Read the model definition and answer for the solid it produces. Units are mm, in the model's axes. A direction names the side the tool comes from. Coordinates: 2 decimals unless noted, no trailing zeros. Loops run counter-clockwise (first coordinate to the right, second up) from the corner with the lowest first, then second, coordinate; pieces in that order, holes last. Notation, with made-up numbers: (58.25, -21) -> (62.25, -21) arc R28 ccw to (62.25, 16) -> close; hole circle Ø3 at (89, 18). An arc over 180 degrees is marked (long way). Answer as a JSON object with one key per item and string values. Group by question number.
Q1. The part is cut by section D-D on x = 95. Write down the section's boundary in (y, z), and give its area (3 significant figures).
Q2. The part is cut by section A-A on x = 26. Write down the section's boundary in (y, z), and give its area (3 significant figures).
Q3. Determine the mould class of faces 5 (the flat face through (0, 3, 40)), 6 (the cylindrical face through (46.69, 3.2, 55.96)), 7 (the flat face through (6, 3, 0)) for opening direction X: released by +X, released by -X, zero draft, split by the parting line, or undercut.
Q4. The part is cut by section B-B on z = 49. Write down the section's boundary in (x, y), and give its area (3 significant figures).
Q5. For faces 1 (the flat face through (112.5, 3, -47)), 2 (the flat face through (122, 3, 0)), 3 (the flat face through (12, 3, 6)), 4 (the flat face through (63, 6.5, 13)), determine the directions among +Z, -Z, +X, -X, +Y, -Y from which every point of the face is accessible in a straight line to the end or side of a thin tool.
Q6. Straight lines are drawn through the part: line 1 along X through (y, z) = (5, 61); line 2 along Z through (x, y) = (37.5, 2); line 3 along Z through (x, y) = (36.5, 5.25). For each, find the intervals that lie inside material, in ascending order. Write a range as [from, to].
Q7. The part is cut by section C-C on y = 1. Write down the section's boundary in (x, z).
Q8. Each of these flat-tipped pins is pushed along its axis until it touches: P1, Ø1.8, axis at x = 120.5, y = 2.5, coming from the +Z side; P2, Ø3, axis at x = 4, y = 2, coming from the +Z side; P3, Ø2, axis at y = 2, z = 19.5, coming from the -X side; P4, Ø3, axis at y = 3.5, z = 9.5, coming from the +X side. Where does it stop, or does it pass through?
Autodesk Inventor part; units mm, degrees
ref_plane "YZ Plane" through (0, 0, 0) normal (1, 0, 0) x (0, 1, 0)
ref_plane "XZ Plane" through (0, 0, 0) normal (0, 1, 0) x (-1, 0, 0)
ref_plane "XY Plane" through (0, 0, 0) normal (0, 0, 1) x (1, 0, 0)
sketch "Sketch1" plane through (0, 0, 0) normal (0, 1, 0) x (-1, 0, 0)
  line L0 (0, -6) -> (0, 0)
  line L1 (0, 0) -> (-12, 0)
  line L2 (-12, 0) -> (-12, 13)
  line L3 (-12, 13) -> (0, 13)
  line L4 (0, 13) -> (0, 67)
  line L5 (0, 67) -> (-8, 75)
  line L6 (-8, 75) -> (-67, 75)
  line L7 (-67, 75) -> (-75, 67)
  line L8 (0, -6) -> (-100, -50)
  line L9 (-100, -50) -> (-124.5, -50)
  line L10 (-124.5, -50) -> (-124.5, 0)
  line L11 (-124.5, 0) -> (-118.5, 0)
  line L12 (-118.5, 0) -> (-118.5, 13)
  line L13 (-118.5, 13) -> (-124.5, 13)
  line L14 (-124.5, 13) -> (-124.5, 19)
  line L15 (-124.5, 19) -> (-75, 19)
  line L16 (-75, 19) -> (-75, 67)
  circle A0 centre (-26, 55) radius 4
  circle A1 centre (-49, 55) radius 2.5
  line L17 (-106, -50) -> (-112.5, -50) construction
  line L18 (-112.5, -50) -> (-112.5, 13) construction
  line L19 (-112.5, 13) -> (-106, 13) construction
  line L20 (-106, 13) -> (-106, -50) construction
  dimension "d0" = 13
  dimension "d1" = 12
  dimension "d2" = 6
  dimension "d3" = 6
  dimension "d4" = 6
  dimension "d6" = 75
  dimension "d7" = 8
  dimension "d8" = 5
  dimension "d9" = 23
  dimension "d10" = 106.5
  dimension "d11" = 45
  dimension "d12" = 8
  dimension "d13" = 6.5
  dimension "d14" = 6
  dimension "d15" = 6
  dimension "d16" = 42
  dimension "d17" = 20
  dimension "d18" = 50
  dimension "d19" = 26
extrude "Extrusion1" add sketch "Sketch1" along normal blind 6.5
sketch "Sketch3" plane through (0, 6.5, 0) normal (0, 1, 0) x (1, 0, 0)
  line L0 (124.5, 0) -> (124.5, 50)
  line L1 (124.5, 50) -> (100, 50)
  line L2 (106, 50) -> (112.5, 50)
  line L3 (112.5, 50) -> (112.5, 44)
  line L4 (112.5, 44) -> (106, 44)
  line L5 (106, 44) -> (106, 50)
  dimension "d27" = 6
  dimension "d28" = 6.5
  dimension "d29" = 12
extrude "Extrusion3" cut sketch "Sketch3" against normal through all
chamfer "Chamfer1" distance 2 angle 45 3 edges at (75, 3.25, 19) (124.5, 3.25, 19) (124.5, 3.25, -50)
sketch "Sketch4" plane through (0, 6.5, 0) normal (0, 1, 0) x (1, 0, 0)
  line L0 (124.5, 0) -> (124.5, 48)
  circle A0 centre (26, -55) radius 4
  circle A1 centre (49, -55) radius 2.5
  circle A2 centre (37.5, -49) radius 2.25
  circle A3 centre (37.5, -61) radius 2.25
  line L1 (37.5, -49) -> (37.5, -61) construction
  line L2 (26, -55) -> (49, -55) construction
  point P0 (37.5, -55)
  dimension "d35" = 12
  dimension "d36" = 4.5
extrude "Extrusion4" cut sketch "Sketch4" against normal through all contours A2 | A3
equation "\"d2\" = d3"
equation "\"d4\" = d3"
properties part number "z_axis_top"
Final values:
{
 "1": {"outline": "(0, -47.8) -> (6.5, -47.8) -> (6.5, 19) -> (0, 19) -> close", "area": "434 mm2"},
 "2": {"outline": "(0, -17.44) -> (6.5, -17.44) -> (6.5, 51) -> (0, 51) -> close; (0, 59) -> (6.5, 59) -> (6.5, 75) -> (0, 75) -> close", "area": "549 mm2"},
 "3": {"face 5": "released by -X", "face 6": "undercut", "face 7": "zero draft"},
 "4": {"outline": "(0, 0) -> (35.25, 0) -> (35.25, 6.5) -> (0, 6.5) -> close; (39.75, 0) -> (75, 0) -> (75, 6.5) -> (39.75, 6.5) -> close", "area": "458 mm2"},
 "5": {"face 1": "-Z, +Y, -Y", "face 2": "+X, +Y, -Y", "face 3": "-X, +Y, -Y", "face 4": "+Z, -Z, +X, -X, +Y"},
 "6": {"line 1": "x = [0, 35.25], [39.75, 75]", "line 2": "z = [-22.5, 46.75], [51.25, 58.75], [63.25, 75]", "line 3": "z = [-22.06, 46.98], [51.02, 58.98], [63.02, 75]"},
 "7": {"outline": "(0, -6) -> (100, -50) -> (106, -50) -> (106, -44) -> (112.5, -44) -> (112.5, -50) -> (122.5, -50) -> (124.5, -48) -> (124.5, 0) -> (118.5, 0) -> (118.5, 13) -> (124.5, 13) -> (124.5, 17) -> (122.5, 19) -> (77, 19) -> (75, 21) -> (75, 67) -> (67, 75) -> (8, 75) -> (0, 67) -> (0, 13) -> (12, 13) -> (12, 0) -> (0, 0) -> close; hole circle Ø8 at (26, 55); hole circle Ø4.5 at (37.5, 49); hole circle Ø4.5 at (37.5, 61); hole circle Ø5 at (49, 55)"},
 "8": {"P1": "stops at z = 19", "P2": "stops at z = 72.5", "P3": "stops at x = 0", "P4": "stops at x = 118.5"}
}
